```python
from build123d import *

# Parameters (mm, degrees)
ESQUISSE1_W             = 120
ESQUISSE1_H             = 80
BOSS_EXTRU_1_DEPTH      = 5
ESQUISSE2_R             = 1.6
ENL_V_MAT_EXTRU_3_DEPTH = 10


with BuildPart() as part:
    # Esquisse1 → Boss.-Extru.1 (new body)
    with BuildSketch(Plane(origin=(0, 0, 0), x_dir=(1, 0, 0), z_dir=(0, 1, 0))):
        with Locations((60, 40)):
            Rectangle(ESQUISSE1_W, ESQUISSE1_H)
    extrude(amount=BOSS_EXTRU_1_DEPTH)

    # Esquisse2 → Enlèv. mat.-Extru.3 (cut)
    with BuildSketch(Plane(origin=(0, 0, 0), x_dir=(1, 0, 0), z_dir=(0, 1, 0))):
        with Locations(Location((5, 75, 0), (0, 0, 90))):
            Circle(ESQUISSE2_R)
        with Locations(Location((115, 75, 0), (0, 0, 90))):
            Circle(ESQUISSE2_R)
        with Locations(Location((115, 5, 0), (0, 0, 90))):
            Circle(ESQUISSE2_R)
        with Locations(Location((5, 5, 0), (0, 0, 90))):
            Circle(ESQUISSE2_R)
    extrude(amount=ENL_V_MAT_EXTRU_3_DEPTH, mode=Mode.SUBTRACT)


solid = part.part
```
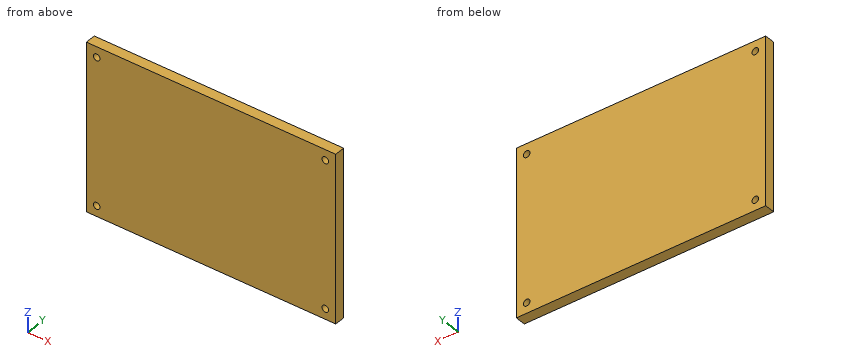
Source: CAD feature listing. Evaluate the final solid. Frame: model axes, mm. Round coordinates to 2 decimals unless told otherwise and drop trailing zeros. Loops run counter-clockwise (first coordinate to the right, second up) from the corner with the lowest first, then second, coordinate; pieces in that order, holes last.
(1) Section query B-B (x = 5). Output: boundary loops of the cut face in (y, z).
From the geometry:
outline: (0, -80) - (5, -80) - (5, -76.6) - (0, -76.6) - close; (0, -73.4) - (5, -73.4) - (5, -6.6) - (0, -6.6) - close; (0, -3.4) - (5, -3.4) - (5, 0) - (0, 0) - close
(2) Section query A-A (z = -75). Output: boundary loops of the cut face in (x, y), and give its area (3 significant figures).
From the geometry:
outline: (0, 0) - (3.4, 0) - (3.4, 5) - (0, 5) - close; (6.6, 0) - (113.4, 0) - (113.4, 5) - (6.6, 5) - close; (116.6, 0) - (120, 0) - (120, 5) - (116.6, 5) - close
area: 568 mm2
(3) Material intervals for probe 1 along X at (y, z) = (2.2, -75); probe 2 along Z at (x, y) = (5, 2.6); probe 3 along X at (y, z) = (3.85, -74.5), sorted ascending.
From the geometry:
probe 1: x = 0 to 3.4, 6.6 to 113.4, 116.6 to 120
probe 2: z = -80 to -76.6, -73.4 to -6.6, -3.4 to 0
probe 3: x = 0 to 3.48, 6.52 to 113.48, 116.52 to 120
(4) Contact query for a flat-ended pin moving along its axis: pin 1 Ø2.5 at (x, z) = (115, -5) entering from -Y. Output: stop coordinate, or through.
From the geometry:
pin 1: passes through
